For this review, take the finished solid that the model builds, in its own axes (mm). Face numbers are marked on the shaded views. A direction names the side the tool comes from. Coordinates: 2 decimals unless noted, no trailing zeros. Loops run counter-clockwise (first coordinate to the right, second up) from the corner with the lowest first, then second, coordinate; pieces in that order, holes last. Notation, with made-up numbers: (41.5, 65.5) -> (80.5, 65.5) arc R21 ccw to (80.5, 78.5) -> close; hole circle Ø11 at (45.25, 3). An arc over 180 degrees is marked (long way). Use a Markdown table: item, result.
from build123d import *

# Parameters (mm, degrees)
BOSS_EXTRUDE1_DEPTH     = 50.8
CUT_EXTRUDE1_DEPTH      = 147.463544952
CUT_EXTRUDE1_DEPTH_BACK = 147.463544952
FILLET1_R               = 6.35
SKETCH5_W               = 19.05
SKETCH5_H               = 19.05
SKETCH5_W_2             = 47.515662577
CUT_EXTRUDE2_DEPTH      = 147.463544952
SKETCH6_R               = 12.7
CUT_EXTRUDE3_DEPTH      = 131.754502791
SKETCH7_R               = 15.875
SKETCH7_R_2             = 6.35
CUT_EXTRUDE4_DEPTH      = 125.595997127
SKETCH8_R               = 11.1125
CUT_EXTRUDE5_DEPTH      = 6.35


with BuildPart() as part:
    # Sketch2 → Boss-Extrude1 (new body)
    with BuildSketch(Plane(origin=(0, 0, 0), x_dir=(1, 0, 0), z_dir=(0, 1, 0))):
        with BuildLine():
            Line((0, -38.1), (114.3, -38.1))
            Line((114.3, -38.1), (114.3, 38.1))
            Line((114.3, 38.1), (0, 38.1))
            ThreePointArc((0, 38.1), (-38.1, 0), (0, -38.1))
        make_face()
    extrude(amount=BOSS_EXTRUDE1_DEPTH)

    # Sketch3 → Cut-Extrude1 (cut, two sides: drawn at the far end of the back side and taken through both)
    with BuildSketch(Plane.XY.offset(38.1).offset(-CUT_EXTRUDE1_DEPTH_BACK)):
        Polygon((38.1, 372.144327072), (38.1, 50.8), (38.1, 31.75), (114.3, 31.75), (435.644327072, 31.75), (853.647106265, 519.932735), (456.102779193, 860.327062073), align=None)
    extrude(amount=CUT_EXTRUDE1_DEPTH + CUT_EXTRUDE1_DEPTH_BACK, mode=Mode.SUBTRACT)

    # Fillet1
    fillet1_edges = [part.edges().sort_by_distance(p)[0] for p in [
        (38.1, 31.75, 0),
    ]]
    fillet(fillet1_edges, radius=FILLET1_R)

    # Sketch5 → Cut-Extrude2 (cut, through all)
    with BuildSketch(Plane.XY.offset(38.1)):
        with Locations((9.525, 25.4)):
            Rectangle(SKETCH5_W, SKETCH5_H)
        with Locations((-23.757831289, 25.4)):
            Rectangle(SKETCH5_W_2, SKETCH5_H)
    extrude(amount=-CUT_EXTRUDE2_DEPTH, mode=Mode.SUBTRACT)

    # Sketch6 → Cut-Extrude3 (cut, through all)
    with BuildSketch(Plane(origin=(0, 50.8, 0), x_dir=(1, 0, 0), z_dir=(0, 1, 0))):
        with Locations(Location((0, 0, 0), (0, 0, 270))):
            Circle(SKETCH6_R)
    extrude(amount=-CUT_EXTRUDE3_DEPTH, mode=Mode.SUBTRACT)

    # Sketch7 → Cut-Extrude4 (cut, through all)
    with BuildSketch(Plane(origin=(0, 31.75, 0), x_dir=(1, 0, 0), z_dir=(0, 1, 0))):
        with Locations((114.3, 0)):
            Circle(SKETCH7_R)
        with Locations(Location((69.85, 0, 0), (0, 0, 270))):
            Circle(SKETCH7_R_2)
    extrude(amount=-CUT_EXTRUDE4_DEPTH, mode=Mode.SUBTRACT)

    # Sketch8 → Cut-Extrude5 (cut)
    with BuildSketch(Plane(origin=(0, 31.75, 0), x_dir=(1, 0, 0), z_dir=(0, 1, 0))):
        with Locations(Location((69.85, 0, 0), (0, 0, 270))):
            Circle(SKETCH8_R)
    extrude(amount=-CUT_EXTRUDE5_DEPTH, mode=Mode.SUBTRACT)


solid = part.part
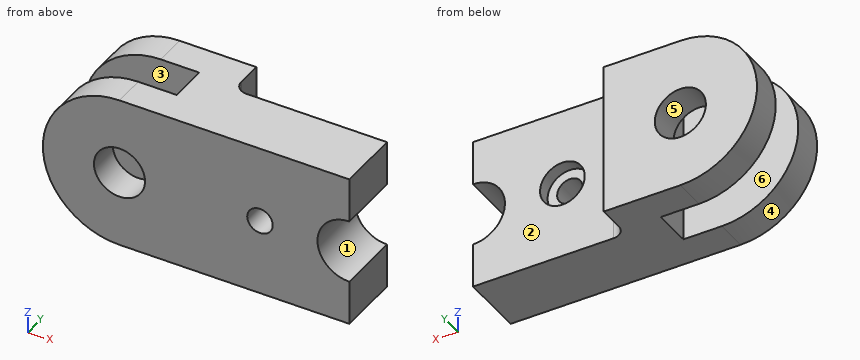
(1) Take a section at B-B on x = 69.85. Write out the cut boundary in (y, z), plus the area to 3 significant figures.
Found:
| item | result |
|---|---|
| outline | (0, -38.1) -> (31.75, -38.1) -> (31.75, -11.11) -> (25.4, -11.11) -> (25.4, -6.35) -> (0, -6.35) -> close; (0, 6.35) -> (25.4, 6.35) -> (25.4, 11.11) -> (31.75, 11.11) -> (31.75, 38.1) -> (0, 38.1) -> close |
| area | 1,960 mm^2 |
(2) For line 1 along X through (y, z) = (15.75, 0) (3 decimals); line 2 along Y through (x, z) = (-30, -21.5) (3 decimals); line 3 along X through (y, z) = (12.5, 3), list the stretches that pass through material, from the lowest coordinate up.
Found:
| item | result |
|---|---|
| line 1 | x = -38.1 to -12.7, 12.7 to 63.5, 76.2 to 98.425 |
| line 2 | y = 0 to 15.875, 34.925 to 50.8 |
| line 3 | x = -37.98 to -12.34, 12.34 to 64.25, 75.45 to 98.71 |
(3) For the marked faces 1, 2 and 3, list the 3-axis set-ups (+Z, -Z, +X, -X, +Y, -Y) from which the entire face can be reached by the end or side of a thin tool; tool diameter is ignored.
Found:
| item | result |
|---|---|
| face 1 | +X, +Y, -Y |
| face 2 | +Z, -Z, +X, +Y |
| face 3 | +Z, -Z, -X |
(4) Mouldability with a two-part tool opening along Z and no side actions: class the marked faces 4, 5 and 6 as pulls with the +Z half, pulls with the -Z half, needs draft (parallel to the pull), parting line crosses it, or undercut.
Found:
| item | result |
|---|---|
| face 4 | parting line crosses it |
| face 5 | undercut |
| face 6 | needs draft |
(5) Take a section at A-A on z = 0. State how many separate pieces and enclosed holes the cut face has, plus the area to 3 significant figures.
Found:
| item | result |
|---|---|
| separate pieces | 4 |
| enclosed holes | 0 |
| area | 3,440 mm^2 |
(6) For pin 1 Ø9.5 at (y, z) = (30, 5.5) entering from -X; pin 2 Ø2 at (x, z) = (83.5, 18) entering from +Y; pin 3 Ø1.5 at (x, z) = (52.5, 14.5) entering from -Y; pin 4 Ø10 at (y, z) = (44.5, 7.5) entering from +X, all flat-tipped, find the tip position at first contact; note any pin that passes through.
Found:
| item | result |
|---|---|
| pin 1 | stops at x = 19.05 |
| pin 2 | stops at y = 31.75 |
| pin 3 | stops at y = 0 |
| pin 4 | stops at x = 38.1 |
(7) Take a section at D-D on x = -9.5. Write out the cut boundary in (y, z) (3 decimals).
Found:
| item | result |
|---|---|
| outline | (0, -36.897) -> (15.875, -36.897) -> (15.875, -8.429) -> (0, -8.429) -> close; (0, 8.429) -> (15.875, 8.429) -> (15.875, 36.897) -> (0, 36.897) -> close; (34.925, -36.897) -> (50.8, -36.897) -> (50.8, -8.429) -> (34.925, -8.429) -> close; (34.925, 8.429) -> (50.8, 8.429) -> (50.8, 36.897) -> (34.925, 36.897) -> close |
(8) Take a section at C-C on y = 23. Write out the cut boundary in (x, z) (3 decimals), plus the area to 3 significant figures.
Found:
| item | result |
|---|---|
| outline | (19.05, -38.1) -> (114.3, -38.1) -> (114.3, -15.875) arc R15.875 cw to (114.3, 15.875) -> (114.3, 38.1) -> (19.05, 38.1) -> close; hole circle Ø12.7 at (69.85, 0) |
| area | 6,740 mm^2 |
